Input: dimensioned drawing with shaded views. Units: mm. Origin: part minimum x, y, z. Give positions to 0.01 mm unless a question says otherwise; leave off trailing zeros. Write each loop counter-clockwise with the first axis right and the second up, starting at its lowest first coordinate (ties: lowest second). Pieces come first, ordered by that corner, then holes.
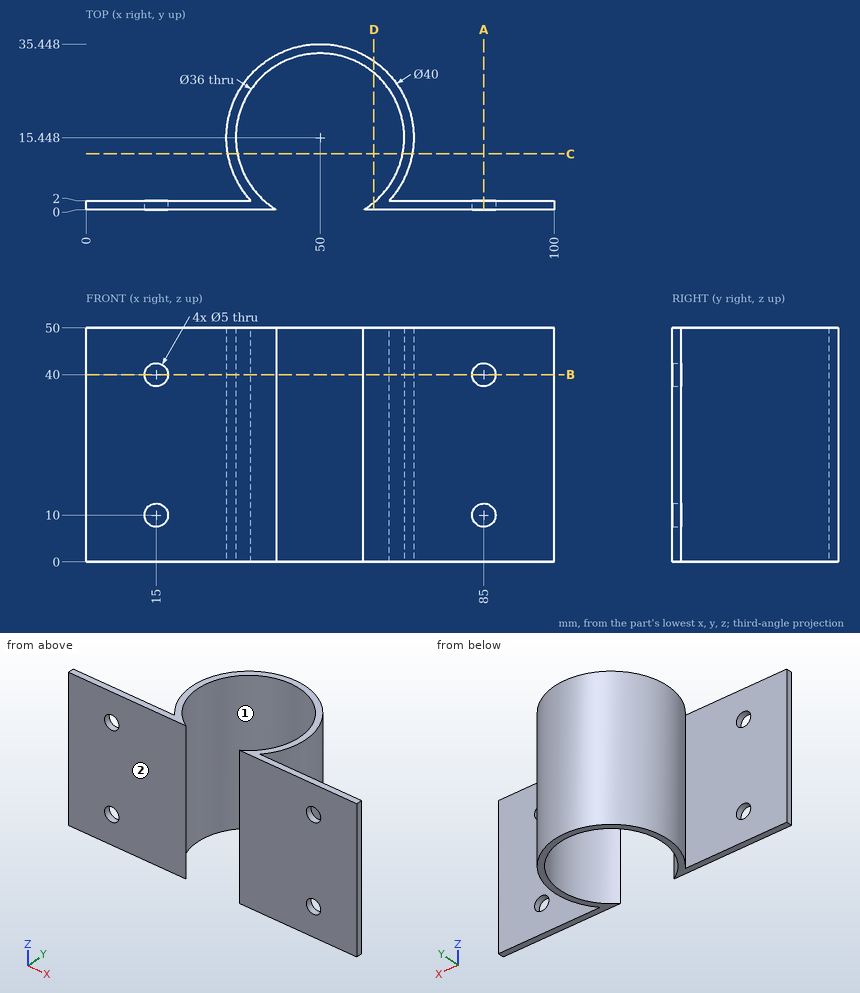
Item 1: Section C-C, the plane y = 12. Return the cut outline in (x, z).
Found:
outline: (30.3, 0) - (32.33, 0) - (32.33, 50) - (30.3, 50) - close; (67.67, 0) - (69.7, 0) - (69.7, 50) - (67.67, 50) - close
Item 2: Section B-B, the plane z = 40. Return the cut outline in (x, y).
Found:
outline: (0, 0) - (12.5, 0) - (12.5, 2) - (0, 2) - close; (17.5, 0) - (40.76, 0) arc R18 cw (long way) to (59.24, 0) - (82.5, 0) - (82.5, 2) - (64.8, 2) arc R20 ccw (long way) to (35.2, 2) - (17.5, 2) - close; (87.5, 0) - (100, 0) - (100, 2) - (87.5, 2) - close
Item 3: Section D-D, the plane x = 61.5. Return the cut outline in (y, z) (1 decimal), plus the area to 3 significant figures.
Found:
outline: (0, 0) - (1.6, 0) - (1.6, 50) - (0, 50) - close; (29.3, 0) - (31.8, 0) - (31.8, 50) - (29.3, 50) - close
area: 206 mm2
Item 4: Section A-A, the plane x = 85. Return the cut outline in (y, z).
Found:
outline: (0, 0) - (2, 0) - (2, 7.5) - (0, 7.5) - close; (0, 12.5) - (2, 12.5) - (2, 37.5) - (0, 37.5) - close; (0, 42.5) - (2, 42.5) - (2, 50) - (0, 50) - close
Item 5: Pull-direction query (X, two-part tool) for the marked faces 1 and 2; classes: +X half, -X half, draft (parallel to the pull), parting line (faces both ways), or undercut.
Found:
face 1: undercut
face 2: draft
Item 6: Line query: L1, parallel to Z at x = 85, y = 0.9; L2, parallel to X at y = 15, z = 16 (1 decimal); L3, parallel to X at y = 0.4, z = 10 (1 decimal). Output: solid intervals per line, ascending.
Found:
L1: z = 0 to 7.5, 12.5 to 37.5, 42.5 to 50
L2: x = 30 to 32, 68 to 70
L3: x = 0 to 12.5, 17.5 to 40.1, 59.9 to 82.5, 87.5 to 100
Item 7: Pin query (flat end, axial travel): pin 1 Ø6 at (x, z) = (85, 40) entering from +Y; pin 2 Ø2 at (y, z) = (18.5, 27) entering from +X (1 decimal). Return the tip coordinate at first contact, or that it passes through.
Found:
pin 1: stops at y = 2
pin 2: stops at x = 69.9
